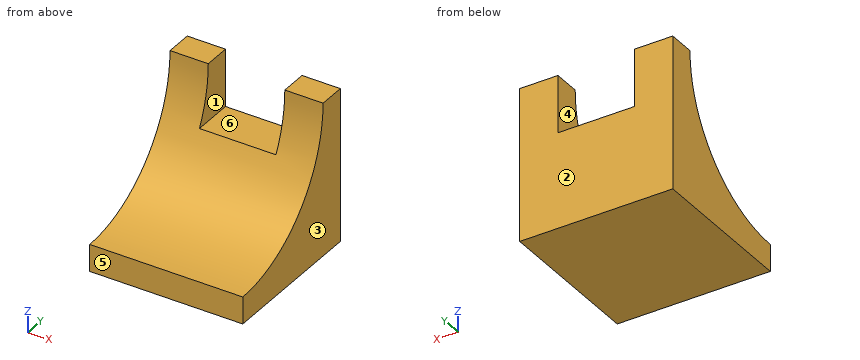
from build123d import *

# Parameters (mm, degrees)
F1_DEPTH = 40
F3_DEPTH = 80.001


with BuildPart() as f1:
    # F0 (on Front) → F1 (new body, symmetric)
    with BuildSketch(Plane.XZ):
        Polygon((-21.581216, 48.518489), (-41.581216, 48.518489), (-41.581216, -31.481511), (38.418784, -31.481511), (38.418784, 48.518489), (18.418784, 48.518489), (18.418784, 18.518489), (-21.581216, 18.518489), align=None)
    extrude(amount=F1_DEPTH, both=True)

    # F2 (on face) → F3 (cut, through all)
    with BuildSketch(Plane(origin=(-41.581216, 0, 0), x_dir=(0, -1, 0), z_dir=(-1, 0, 0))):
        with BuildLine():
            Line((40, -17.350387), (40, -15.578494))
            Line((40, -15.578494), (40, 48.518489))
            Line((40, 48.518489), (-25.868876, 48.518489))
            ThreePointArc((-25.868876, 48.518489), (-6.576329, 1.94216), (40, -17.350387))
        make_face()
    extrude(amount=-F3_DEPTH, mode=Mode.SUBTRACT)


solid = f1.part
Read the model definition and answer for the solid it produces. Units are mm, in the model's axes. Face numbers are marked on the shaded views. A direction names the side the tool comes from. Give positions to 0.01 mm unless a question says otherwise; leave off trailing zeros. Write each loop counter-clockwise with the first axis right and the second up, starting at its lowest first coordinate (ties: lowest second). Pieces come first, ordered by that corner, then holes. Notation, with made-up numbers: (-19.75, 60.25) - (25.25, 60.25) arc R16 cw to (25.25, 65.25) - close; hole circle Ø1 at (-16, 3.5). An arc over 180 degrees is marked (long way). Return JSON: item names as keys, results as strings.
Q1. For a pull along X with two mould halves and no side action, classify the marked faces 1, 2, 3 and 4 as released by +X, released by -X, zero draft, split by the parting line, or undercut.
Reply:
{"face 1": "undercut", "face 2": "zero draft", "face 3": "released by +X", "face 4": "undercut"}
Q2. A cutting plane is placed at A-A, the plane z = 25.5. Determine the outline of the cut face in (x, y).
Reply:
{"outline": "(-41.58, 21.72) - (-21.58, 21.72) - (-21.58, 40) - (-41.58, 40) - close; (18.42, 21.72) - (38.42, 21.72) - (38.42, 40) - (18.42, 40) - close"}
Q3. For the marked faces 5 and 6, determine the directions among +Z, -Z, +X, -X, +Y, -Y from which every point of the face is accessible in a straight line to the end or side of a thin tool.
Reply:
{"face 5": "+Z, -Z, +X, -X, -Y", "face 6": "+Z, +Y, -Y"}
Q4. A cutting plane is placed at D-D, the plane x = 15. Determine the outline of the cut face in (y, z).
Reply:
{"outline": "(-40, -31.48) - (40, -31.48) - (40, 18.52) - (18.64, 18.52) arc R65.87 cw to (-40, -17.35) - close"}
Q5. A cutting plane is placed at C-C, the plane x = -36. Determine the outline of the cut face in (y, z).
Reply:
{"outline": "(-40, -31.48) - (40, -31.48) - (40, 48.52) - (25.87, 48.52) arc R65.87 cw to (-40, -17.35) - close"}
Q6. A cutting plane is placed at B-B, the plane y = 28.5. Determine the outline of the cut face in (x, z).
Reply:
{"outline": "(-41.58, -31.48) - (38.42, -31.48) - (38.42, 48.52) - (18.42, 48.52) - (18.42, 18.52) - (-21.58, 18.52) - (-21.58, 48.52) - (-41.58, 48.52) - close"}
Q7. Consider line 1 along X through (y, z) = (29.5, 29); line 2 along Z through (x, y) = (-9.5, 31); line 3 along Z through (x, y) = (-21.5, -14). Determine where each line is inside the solid, lowest interval first. Write a range as [from, to].
Reply:
{"line 1": "[-41.58, -21.58], [18.42, 38.42]", "line 2": "[-31.48, 18.52]", "line 3": "[-31.48, -12]"}
Q8. Given P1, Ø10.5, axis at x = -3, y = 29, coming from the +Z side; P2, Ø8, axis at y = 19.5, z = 37.5, coming from the -X side, each flat-ended and moving along its own axis, determine where each tip first touches the part or whether it passes through.
Reply:
{"P1": "z = 18.52", "P2": "through"}
